Verification items for the finished model (mm, model axes). Face numbers are marked on the shaded views. A direction names the side the tool comes from. Coordinates: 2 decimals unless noted, no trailing zeros. Loops run counter-clockwise (first coordinate to the right, second up) from the corner with the lowest first, then second, coordinate; pieces in that order, holes last. Notation, with made-up numbers: (72, -4.5) -> (126, -4.5) arc R13 ccw to (126, 2.5) -> close; hole circle Ø2 at (-6.5, 1). An arc over 180 degrees is marked (long way). Write item = value, one per line.
```python
from build123d import *

# Parameters (mm, degrees)
SKETCH1_R           = 15
BOSS_EXTRUDE1_DEPTH = 15
SKETCH2_R           = 1.45
BOSS_EXTRUDE2_DEPTH = 15
BOSS_EXTRUDE3_DEPTH = 3
SKETCH5_R           = 1.5
CUT_EXTRUDE1_DEPTH  = 113.467773162
FILLET1_R           = 5


with BuildPart() as part:
    # Sketch1 → Boss-Extrude1 (new body)
    with BuildSketch(Plane.XY):
        Circle(SKETCH1_R)
    extrude(amount=BOSS_EXTRUDE1_DEPTH)

    # Sketch2 → Boss-Extrude2 (add)
    with BuildSketch(Plane.XY.offset(15)):
        Circle(SKETCH2_R)
    extrude(amount=BOSS_EXTRUDE2_DEPTH)

    # Sketch4 → Boss-Extrude3 (add)
    with BuildSketch(Plane.XY.offset(15)):
        with BuildLine():
            Line((5, -10), (7.465093605, -6.653749128))
            ThreePointArc((7.465093605, -6.653749128), (0, 10), (-7.465093605, -6.653749128))
            Line((-7.465093605, -6.653749128), (-5, -10))
            Line((-5, -10), (-5, -110))
            Line((-5, -110), (5, -110))
            Line((5, -110), (5, -10))
        make_face()
    extrude(amount=BOSS_EXTRUDE3_DEPTH)

    # Sketch5 → Cut-Extrude1 (cut, through all)
    with BuildSketch(Plane.XY.offset(18)):
        with Locations((0, -105)):
            Circle(SKETCH5_R)
    extrude(amount=-CUT_EXTRUDE1_DEPTH, mode=Mode.SUBTRACT)

    # Fillet1
    fillet1_edges = [part.edges().sort_by_distance(p)[0] for p in [
        (5, -10, 16.5),
        (-5, -10, 16.5),
        (-5, -110, 16.5),
        (5, -110, 16.5),
    ]]
    fillet(fillet1_edges, radius=FILLET1_R - 0.0001)  # a hair under: the kernel refuses the full size


solid = part.part
```
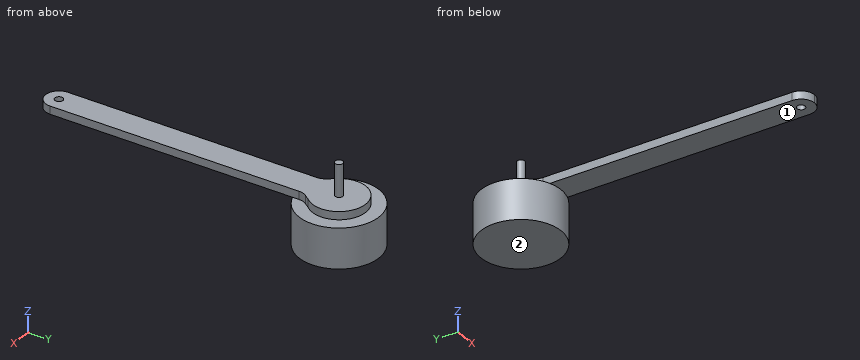
1) Sectioned sample at A-A, the plane y = 0. Record the cut outline in (x, z), plus the area to 3 significant figures.
Ans:
outline = (-15, 0) -> (15, 0) -> (15, 15) -> (10, 15) -> (10, 18) -> (1.45, 18) -> (1.45, 30) -> (-1.45, 30) -> (-1.45, 18) -> (-10, 18) -> (-10, 15) -> (-15, 15) -> close
area = 545 mm2
2) Depth check by flat-ended pin: pin 1 Ø4 at (x, y) = (0, -105) entering from -Z; pin 2 Ø3 at (y, z) = (-89, 16) entering from -X; pin 3 Ø6 at (x, y) = (-2.5, -54.5) entering from +Z; pin 4 Ø4 at (x, z) = (7.5, 21.5) entering from -Y. Enter the tip coordinate at first touch or a pass-through.
Ans:
pin_1 = 15
pin_2 = -5
pin_3 = 18
pin_4 = through
3) Tool access check on the marked faces 1 and 2. Record the directions out of +Z, -Z, +X, -X, +Y, -Y that give a thin tool (end or side, any length) a straight path to the whole face; none if there is none.
Ans:
face_1 = -Z, +X, -X, -Y
face_2 = -Z, +X, -X, +Y, -Y
4) Sectioned sample at B-B, the plane z = 10.75. Record the cut outline in (x, y).
Ans:
outline = circle Ø30 at (0, 0)
5) Sectioned sample at C-C, the plane x = -12.25. Record the cut outline in (y, z), plus the area to 3 significant figures.
Ans:
outline = (-8.66, 0) -> (8.66, 0) -> (8.66, 15) -> (-8.66, 15) -> close
area = 260 mm2
6) Material ranges on line 1 (X direction, y = -105, z = 15.85); line 2 (Y direction, x = 0, z = 15.95); line 3 (Z direction, x = -13.5, y = 6), recorded low to high.
Ans:
line_1 = -5 to -1.5, 1.5 to 5
line_2 = -110 to -106.5, -103.5 to 10
line_3 = 0 to 15
7) Sectioned sample at D-D, the plane z = 27.5. Record the cut outline in (x, y).
Ans:
outline = circle Ø2.9 at (0, 0)
